Print and shaded views of the part. All mm, measured from the part's lowest x, y and z. Give positions to 0.01 mm unless a question says otherwise; leave off trailing zeros. Loops run counter-clockwise (first coordinate to the right, second up) from the corner with the lowest first, then second, coordinate; pieces in that order, holes last. Notation, with made-up numbers: M 85.5,20 L 118.5,20 A21 cw 118.5,37 Z; hole C 24.5,60.25 d9. An arc over 180 degrees is marked long. Put each result on its own line as item: value. Start each with the question number.
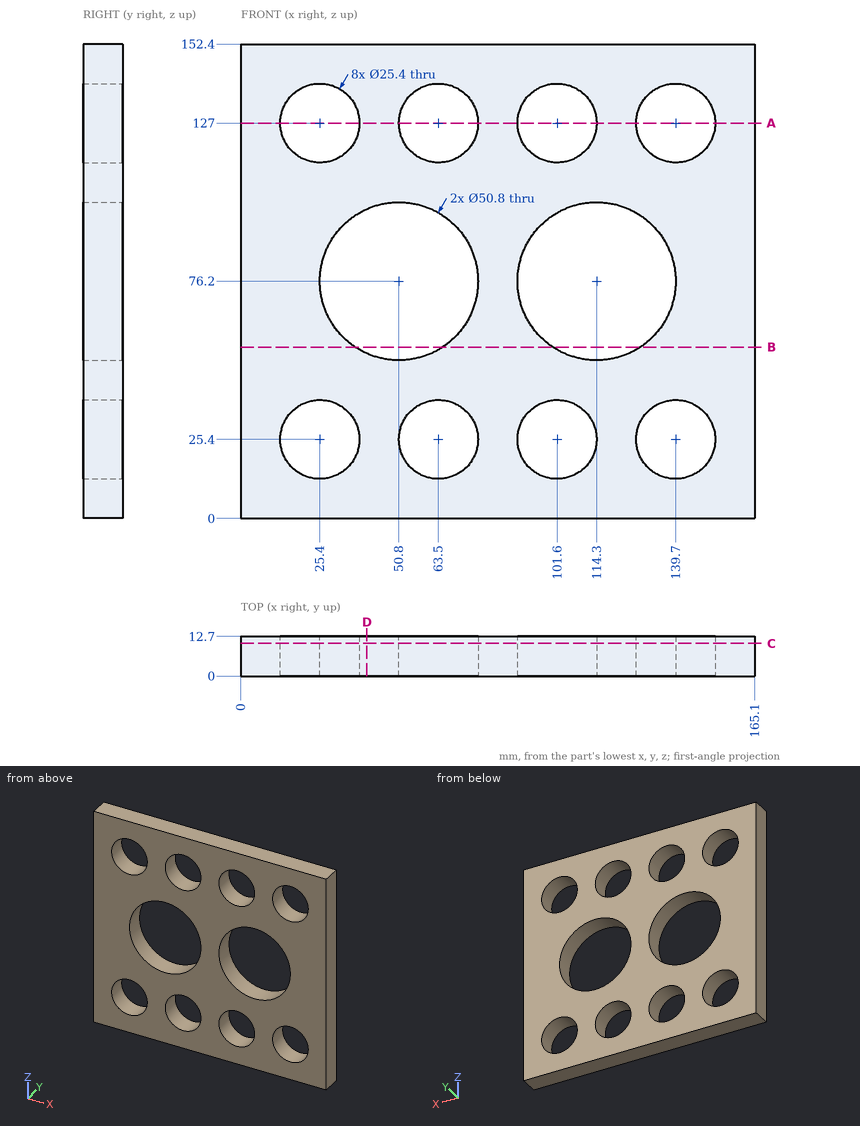
1) Band-saw the part on A-A on z = 127. Give the cut face in (x, y).
2) Wall check: L1, parallel to X at y = 9.25, z = 76.2; L2, parallel to X at y = 9.5, z = 17; L3, parallel to X at y = 5, z = 16. Give the ranges that are in metal, low to high.
3) Band-saw the part on C-C on y = 10.5. State how many separate pieces and enclosed holes the cut face has, then the cut area to 3 significant figures.
4) Band-saw the part on B-B on z = 55. Give the cut face in (x, y), then the cut area to 3 significant figures.
5) Band-saw the part on D-D on x = 40.5. Give the cut face in (y, z).
6) Pin check, flat tip, straight feed: pin 1 Ø20.5 at (x, z) = (101.6, 25.4) entering from -Y. Stop position of the tip, or through.
Evaluation:
1. outline: M 0,0 L 12.7,0 L 12.7,12.7 L 0,12.7 Z; M 38.1,0 L 50.8,0 L 50.8,12.7 L 38.1,12.7 Z; M 76.2,0 L 88.9,0 L 88.9,12.7 L 76.2,12.7 Z; M 114.3,0 L 127,0 L 127,12.7 L 114.3,12.7 Z; M 152.4,0 L 165.1,0 L 165.1,12.7 L 152.4,12.7 Z
2. L1: 0 to 25.4, 76.2 to 88.9, 139.7 to 165.1
2. L2: 0 to 15.87, 34.93 to 53.97, 73.03 to 92.07, 111.13 to 130.17, 149.23 to 165.1
2. L3: 0 to 16.86, 33.94 to 54.96, 72.04 to 93.06, 110.14 to 131.16, 148.24 to 165.1
3. separate pieces: 1
3. enclosed holes: 10
3. area: 17,100 mm2
4. outline: M 0,0 L 36.81,0 L 36.81,12.7 L 0,12.7 Z; M 64.79,0 L 100.31,0 L 100.31,12.7 L 64.79,12.7 Z; M 128.29,0 L 165.1,0 L 165.1,12.7 L 128.29,12.7 Z
4. area: 1,390 mm2
5. outline: M 0,0 L 12.7,0 L 12.7,52.98 L 0,52.98 Z; M 0,99.42 L 12.7,99.42 L 12.7,152.4 L 0,152.4 Z
6. pin 1: through
